Check sheet for the modelled part. Datum: model origin and axes. Units: mm. A direction names the side the tool comes from. Round coordinates to 2 decimals unless told otherwise and drop trailing zeros. Loops run counter-clockwise (first coordinate to the right, second up) from the corner with the lowest first, then second, coordinate; pieces in that order, holes last. Notation, with made-up numbers: (15, -40) -> (31, -40) arc R21 ccw to (31, -15) -> close; hole circle Ø1 at (50.5, 77). An arc over 180 degrees is marked (long way). One line per question, with ' | ' between items.
```python
from build123d import *

# Parameters (mm, degrees)
BOSS_EXTRUDE1_DEPTH = 6
FILLET1_R           = 1
FILLET2_R           = 1
SKETCH3_W           = 7
SKETCH3_H           = 1.35
BOSS_EXTRUDE2_DEPTH = 1
FILLET4_R           = 0.5
SKETCH4_R           = 0.5
CUT_EXTRUDE1_DEPTH  = 1


with BuildPart() as part:
    # Sketch1 → Boss-Extrude1 (new body)
    with BuildSketch(Plane(origin=(0, 0, 0), x_dir=(1, 0, 0), z_dir=(0, 1, 0))):
        with BuildLine():
            Line((-11.381708203, 10.791631839), (-4.712422066, 22.925104071))
            ThreePointArc((-4.712422066, 22.925104071), (-1.039732152, 26.715438863), (4.050994341, 28.108203315))
            Line((4.050994341, 28.108203315), (23.765326904, 28.108203315))
            ThreePointArc((23.765326904, 28.108203315), (24.68179457, 27.508312073), (24.498700382, 26.428377351))
            Line((24.498700382, 26.428377351), (1.333132609, 1.438138803))
            ThreePointArc((1.333132609, 1.438138803), (0.345199416, -0.135386591), (0, -1.960991017))
            Line((0, -1.960991017), (0, -6))
            Line((0, -6), (-12, -6))
            Line((-12, -6), (-12, 8.383181461))
            ThreePointArc((-12, 8.383181461), (-11.842960924, 9.626455161), (-11.381708203, 10.791631839))
        make_face()
    extrude(amount=BOSS_EXTRUDE1_DEPTH)

    # Fillet1
    fillet1_edges = [part.edges().sort_by_distance(p)[0] for p in [
        (-11.842960924, 6, -9.626455161),
        (-12, 6, -1.191590731),
        (0, 6, 3.980495509),
        (0.345199416, 6, 0.135386591),
        (12.915916496, 6, -13.933258077),
        (24.68179457, 6, -27.508312073),
        (13.908160623, 6, -28.108203315),
        (-1.039732152, 6, -26.715438863),
        (-8.047065134, 6, -16.858367955),
    ]]
    fillet(fillet1_edges, radius=FILLET1_R)

    # Fillet2
    fillet2_edges = [part.edges().sort_by_distance(p)[0] for p in [
        (12.915916496, 0, -13.933258077),
        (0.345199416, 0, 0.135386591),
        (0, 0, 3.980495509),
        (-12, 0, -1.191590731),
        (-11.842960924, 0, -9.626455161),
        (-8.047065134, 0, -16.858367955),
        (-1.039732152, 0, -26.715438863),
        (13.908160623, 0, -28.108203315),
        (24.68179457, 0, -27.508312073),
    ]]
    fillet(fillet2_edges, radius=FILLET2_R)

    # Sketch3 → Boss-Extrude2 (add)
    with BuildSketch(Plane.XY.offset(6)):
        with Locations((-6, 6.675)):
            Rectangle(SKETCH3_W, SKETCH3_H)
    extrude(amount=-BOSS_EXTRUDE2_DEPTH)

    # Fillet4
    fillet4_edges = [part.edges().sort_by_distance(p)[0] for p in [
        (-2.5, 6, 5.5),
        (-9.5, 6, 5.5),
        (-9.5, 7.35, 5.5),
        (-2.5, 7.35, 5.5),
    ]]
    fillet(fillet4_edges, radius=FILLET4_R)

    # Sketch4 → Cut-Extrude1 (cut)
    with BuildSketch(Plane(origin=(0, 0, 5), x_dir=(-1, 0, 0), z_dir=(0, 0, -1))):
        with Locations((7.5, 6.7)):
            Circle(SKETCH4_R)
        with Locations(Location((4.5, 6.7, 0), (0, 0, 180))):
            Circle(SKETCH4_R)
    extrude(amount=-CUT_EXTRUDE1_DEPTH, mode=Mode.SUBTRACT)


solid = part.part
```
(1) Mould release check, pull along Y, two halves, no side actions. Record for faces 3 (the face through (-7.8, 7.1, 5.5)), 4 (the face through (0, 3, 4)), 5 (the face through (14.05, 5.7, -27.82)): +Y half, -Y half, draft (parallel to the pull), parting line (faces both ways), or undercut.
Answer:
face 3: undercut | face 4: draft | face 5: +Y half
(2) Go/stop test with flat-tipped pins: pin 1 (3 mm diameter, centred on x = 1.5, y = 3.5, fed in from -Z); pin 2 (2 mm diameter, centred on x = 20, y = 2, fed in from +Z); pin 3 (4 mm diameter, centred on y = 6, z = -10.5, fed in from +X). Record where each tip stops, or that it passes through.
Answer:
pin 1: stops at z = -28.05 | pin 2: stops at z = -20.5 | pin 3: stops at x = 11.41
(3) Scan lines: probe 1 along Y at (x, z) = (-9, 1); probe 2 along Y at (x, z) = (-7.5, 5.4); probe 3 along Z at (x, y) = (-1, 3.75). Record each from-to range of solid material in increasing order.
Answer:
probe 1: y = 0 to 6 | probe 2: y = 0 to 6.2, 7.2 to 7.35 | probe 3: z = -26.74 to 6
(4) Sectioned sample at A-A, the plane y = 2.75. Record the cut outline in (x, z).
Answer:
outline: (-12, -8.38) arc R5 ccw to (-11.38, -10.79) -> (-4.71, -22.93) arc R10 ccw to (4.05, -28.11) -> (23.77, -28.11) arc R1 ccw to (24.5, -26.43) -> (1.33, -1.44) arc R5 cw to (0, 1.96) -> (0, 6) -> (-12, 6) -> close
(5) Set-up check for faces 1 (the face through (24.675, 2.972, -27.523)), 2 (the face through (-0.301, 0.285, 4.009)): record each of +Z, -Z, +X, -X, +Y, -Y from which the full face is reachable in a straight line by a thin tool's end or side.
Answer:
face 1: +X, +Y, -Y | face 2: +Z, +X, -Y
